```python
from build123d import *

# Parameters (mm, degrees)
F0_W          = 50.8
F0_H          = 50.8
F1_DEPTH      = 44.45
F2_R          = 41.6392932994
F3_DEPTH      = 6.35
F3_DEPTH_BACK = 6.35


with BuildPart() as f1:
    # F0 (on Top) → F1 (new body)
    with BuildSketch(Plane.XY):
        Rectangle(F0_W, F0_H)
    extrude(amount=F1_DEPTH)

    # F2 (on face) → F3 (join, two sides)
    with BuildSketch(Plane.XY.offset(44.45)) as f3_sk:
        Circle(F2_R)
        with BuildLine():
            ThreePointArc((25.4, 13.6763064921), (27.9726476241, 7.0521162896), (28.8479004308, 0))
            ThreePointArc((28.8479004308, 0), (27.9726476241, -7.0521162896), (25.4, -13.6763064921))
            Line((25.4, -13.6763064921), (25.4, -25.4))
            Line((25.4, -25.4), (13.6763064921, -25.4))
            ThreePointArc((13.6763064921, -25.4), (0, -28.8479004308), (-13.6763064921, -25.4))
            Line((-13.6763064921, -25.4), (-25.4, -25.4))
            Line((-25.4, -25.4), (-25.4, -13.6763064921))
            ThreePointArc((-25.4, -13.6763064921), (-28.8479004308, 0), (-25.4, 13.6763064921))
            Line((-25.4, 13.6763064921), (-25.4, 25.4))
            Line((-25.4, 25.4), (-13.6763064921, 25.4))
            ThreePointArc((-13.6763064921, 25.4), (0, 28.8479004308), (13.6763064921, 25.4))
            Line((13.6763064921, 25.4), (25.4, 25.4))
            Line((25.4, 25.4), (25.4, 13.6763064921))
        make_face(mode=Mode.SUBTRACT)
    extrude(amount=-F3_DEPTH)
    extrude(f3_sk.sketch, amount=F3_DEPTH_BACK)


solid = f1.part
```
CAD build for the part. Positions are in the model's coordinates, mm. A direction names the side the tool comes from. Round coordinates to 2 decimals unless told otherwise and drop trailing zeros. Loops run counter-clockwise (first coordinate to the right, second up) from the corner with the lowest first, then second, coordinate; pieces in that order, holes last. Notation, with made-up numbers: M 70.25,31.25 L 127.25,31.25 A35 cw 127.25,68.25 Z; hole C 28,-26.75 d9. An arc over 180 degrees is marked long. Return JSON: item names as keys, results as strings. Group by question number.
(1) Saw through at D-D, the plane y = -20.5. List the corners of the cut face in (x, z).
(2) Saw through at C-C, the plane z = 46. List the corners of the cut face in (x, y).
(3) Wall check: probe 1 along X at (y, z) = (0.5, 40); probe 2 along X at (y, z) = (-3, 43.5); probe 3 along X at (y, z) = (15.5, 28). Give the ranges that are in metal, low to high. Write a range as [from, to].
(4) Mould opens along Y. For faces 3 (the flat face through (9, 28, 50.8)), 4 (the flat face through (25.4, -19, 48)) say: +Y half, -Y half, draft (parallel to the pull), parting line (faces both ways), or undercut.
(5) Tool access for faces 1 (the flat face through (0, 0, 0)), 2 (the flat face through (25.4, 20, 48)): list every direction of +Z, -Z, +X, -X, +Y, -Y with a clear straight run to the whole face (end or side of a thin tool).
(6) Saw through at A-A, the plane z = 40. List the corners of the cut face in (x, y), and give its area (3 significant figures).
(7) Saw through at B-B, the plane x = 0. List the corners of the cut face in (y, z).
(8) Drop flat-ended pins along their axis: P1, Ø2, axis at x = 17, y = 13, coming from the +Z side; P2, Ø2, axis at x = -15.5, z = 26.5, coming from the -Y side; P3, Ø13.5, axis at y = -1.5, z = 27, coming from the -X side. Give the stop position or say it passes through.
Answer list:
{
 "1": {"outline": "M -36.24,38.1 L -25.4,38.1 L -25.4,0 L 25.4,0 L 25.4,38.1 L 36.24,38.1 L 36.24,50.8 L 25.4,50.8 L 25.4,44.45 L -25.4,44.45 L -25.4,50.8 L -36.24,50.8 Z"},
 "2": {"outline": "C 0,0 d83.28; hole M -25.4,-25.4 L -13.68,-25.4 A28.85 ccw 13.68,-25.4 L 25.4,-25.4 L 25.4,-13.68 A28.85 ccw 25.4,13.68 L 25.4,25.4 L 13.68,25.4 A28.85 ccw -13.68,25.4 L -25.4,25.4 L -25.4,13.68 A28.85 ccw -25.4,-13.68 Z"},
 "3": {"probe 1": "[-41.64, -28.84], [-25.4, 25.4], [28.84, 41.64]", "probe 2": "[-41.53, -28.69], [-25.4, 25.4], [28.69, 41.53]", "probe 3": "[-25.4, 25.4]"},
 "4": {"face 3": "draft", "face 4": "undercut"},
 "5": {"face 1": "-Z, +X, -X, +Y, -Y", "face 2": "+Z"},
 "6": {"outline": "C 0,0 d83.28; hole M -25.4,-13.68 L -25.4,13.68 A28.85 ccw Z; hole M -13.68,-25.4 A28.85 ccw 13.68,-25.4 Z; hole M -13.68,25.4 L 13.68,25.4 A28.85 ccw Z; hole M 25.4,-13.68 A28.85 ccw 25.4,13.68 Z", "area": "5,190 mm2"},
 "7": {"outline": "M -41.64,38.1 L -28.85,38.1 L -28.85,50.8 L -41.64,50.8 Z; M -25.4,0 L 25.4,0 L 25.4,44.45 L -25.4,44.45 Z; M 28.85,38.1 L 41.64,38.1 L 41.64,50.8 L 28.85,50.8 Z"},
 "8": {"P1": "z = 44.45", "P2": "y = -25.4", "P3": "x = -25.4"}
}
